Autodesk Inventor part; units mm, degrees
ref_plane "YZ Plane" through (0, 0, 0) normal (1, 0, 0) x (0, 1, 0)
ref_plane "XZ Plane" through (0, 0, 0) normal (0, 1, 0) x (-1, 0, 0)
ref_plane "XY Plane" through (0, 0, 0) normal (0, 0, 1) x (1, 0, 0)
sketch "Sketch1" plane through (0, 0, 0) normal (0, 0, 1) x (1, 0, 0)
  line L0 (0, 0) -> (25.4, 0)
  line L1 (25.4, 0) -> (25.4, 25.4)
  line L2 (25.4, 25.4) -> (0, 25.4)
  line L3 (0, 25.4) -> (0, 0)
  line L4 (3.175, 3.175) -> (22.225, 3.175)
  line L5 (22.225, 3.175) -> (22.225, 22.225)
  line L6 (22.225, 22.225) -> (3.175, 22.225)
  line L7 (3.175, 22.225) -> (3.175, 3.175)
  dimension "d0" = 25.4
  dimension "d1" = 25.4
  dimension "d2" = 19.05
  dimension "d3" = 19.05
  dimension "d4" = 3.175
  dimension "d5" = 3.175
extrude "Extrusion1" add sketch "Sketch1" along normal blind 304.8
sketch "Sketch2" plane through (0, 25.4, 0) normal (0, 1, 0) x (1, 0, 0)
  line L0 (25.4, 0) -> (0, 0)
  line L1 (0, 0) -> (0, -304.8)
  line L2 (25.4, -304.8) -> (0, -304.8)
  line L3 (25.4, 0) -> (25.4, -304.8)
  point P0 (12.7, -292.1)
  point P1 (12.7, -12.7)
  point P2 (12.7, -190.5)
  dimension "d8" = 12.7
  dimension "d9" = 12.7
  dimension "d10" = 12.7
  dimension "d11" = 12.7
  dimension "d32" = 12.7
  dimension "d33" = 114.3
sketch "Sketch3" plane through (25.4, 0, 0) normal (1, 0, 0) x (0, 0, -1)
  line L0 (0, 0) -> (-304.8, 0)
  line L1 (0, 0) -> (0, 25.4)
  point P0 (-38.1, 12.7)
  point P1 (-63.5, 12.7)
  point P2 (-88.9, 12.7)
  dimension "d19" = 12.7
  dimension "d20" = 12.7
  dimension "d21" = 12.7
  dimension "d22" = 38.1
  dimension "d23" = 88.9
  dimension "d24" = 63.5
hole "Hole2" at (25.4, 12.7, 38.1) at (25.4, 12.7, 63.5) at (25.4, 12.7, 88.9) direction (-1, 0, 0) diameter 3.9688 end through all
hole "Hole3" at (12.7, 25.4, 292.1) at (12.7, 25.4, 12.7) at (12.7, 25.4, 190.5) direction (0, -1, 0) diameter 6.35 end through all
sketch "Sketch4" plane through (25.4, 0, 0) normal (1, 0, 0) x (0, 0, -1)
  circle A0 centre (-63.5, 12.7) radius 1.9844
  circle A1 centre (-38.1, 12.7) radius 1.9844
  circle A2 centre (-88.9, 12.7) radius 1.9844
  line L0 (0, 0) -> (0, 25.4)
  line L1 (0, 25.4) -> (-304.8, 25.4)
  line L2 (-304.8, 0) -> (-304.8, 25.4)
  line L3 (0, 0) -> (-304.8, 0)
  point P0 (-171.45, 12.7)
  point P1 (-107.95, 12.7)
  point P2 (-146.05, 12.7)
  dimension "d41" = 133.35
  dimension "d42" = 196.85
  dimension "d43" = 158.75
  dimension "d44" = 12.7
  dimension "d45" = 12.7
  dimension "d46" = 12.7
hole "Hole4" at (25.4, 12.7, 171.45) at (25.4, 12.7, 107.95) at (25.4, 12.7, 146.05) direction (-1, 0, 0) diameter 3.9688 end through all
properties part number "mounting block"
Could you check a few things on this model? Use its own coordinates, in mm. A direction names the side the tool comes from. Round coordinates to 2 decimals unless told otherwise and drop trailing zeros. Loops run counter-clockwise (first coordinate to the right, second up) from the corner with the lowest first, then second, coordinate; pieces in that order, holes last. Notation, with made-up numbers: M 80.5,22.25 L 89.5,22.25 A30 ccw 89.5,44.25 Z; hole C -39,27.5 d11. An arc over 180 degrees is marked long. Write item = value, one per line.
1. I want a section at B-B, the plane z = 12.7. Write out the boundary of the cut face in (x, y) (3 decimals).
Results below:
outline = M 0,0 L 9.525,0 L 9.525,3.175 L 3.175,3.175 L 3.175,22.225 L 9.525,22.225 L 9.525,25.4 L 0,25.4 Z; M 15.875,0 L 25.4,0 L 25.4,25.4 L 15.875,25.4 L 15.875,22.225 L 22.225,22.225 L 22.225,3.175 L 15.875,3.175 Z
2. Thinking about a two-plate mould opening in Z: for faces 1 (the face through (14.63, 1.57, 10.18)), 2 (the face through (22.225, 13, 150)), 3 (the face through (24, 13, 0)), which applies, +Z half, -Z half, draft (parallel to the pull), parting line (faces both ways), or undercut?
Results below:
face_1 = undercut
face_2 = draft
face_3 = -Z half
3. I need wall thicknesses on probe 1 along Y at (x, z) = (23.2, 38.1); probe 2 along Y at (x, z) = (5.75, 175) (3 decimals). Which ranges of each line are inside material? Lowest first, please.
Results below:
probe_1 = 0 to 10.72, 14.68 to 25.4
probe_2 = 0 to 3.175, 22.225 to 25.4
4. Which directions (+Z, -Z, +X, -X, +Y, -Y) give clear straight access to the entire face, cutting with the end or side of a thin tool? Please do faces 4 (the face through (12.56, 1.57, 187.33)), 5 (the face through (3.175, 13, 150)).
Results below:
face_4 = +Y, -Y
face_5 = +Z, -Z
5. I want a section at C-C, the plane z = 69. Write out the boundary of the cut face in (x, y) (3 decimals), and give its area (3 significant figures).
Results below:
outline = M 0,0 L 25.4,0 L 25.4,25.4 L 0,25.4 Z; hole M 3.175,3.175 L 22.225,3.175 L 22.225,22.225 L 3.175,22.225 Z
area = 282 mm²
6. Will this pin go through, and if not, where does the flat tip stop? P1, Ø5, axis at x = 3, z = 179, coming from the -Y side.
Results below:
P1 = 0
7. I want a section at A-A, the plane x = 12.7. Count the separate pieces of the cut face and the enclosed holes in it, and give its area (3 significant figures).
Results below:
separate_pieces = 8
enclosed_holes = 0
area = 1,810 mm²
